The listing builds one solid part. Answer for the finished solid, in the listing's coordinates (mm). Give positions to 0.01 mm unless a question says otherwise; leave off trailing zeros. Loops run counter-clockwise (first coordinate to the right, second up) from the corner with the lowest first, then second, coordinate; pieces in that order, holes last.
Item 1: Consider line 1 along X through (y, z) = (-1.8, 37.5); line 2 along X through (y, z) = (1.7, 82.5); line 3 along Y through (x, z) = (-0.25, 95.5). Determine where each line is inside the solid, lowest interval first.
Item 2: Section A-A, the plane z = 97.5 is taken. Give the vertices of the cut face in (x, y).
Item 3: Section B-B, the plane z = 19 is taken. Give the vertices of the cut face in (x, y).
Item 4: Section C-C, the plane x = 0 is taken. Give the number of separate pieces and of enclosed holes in the cut face, and give its area (3 significant figures).
Item 5: This flat-tipped pin is pushed along its axis until it touches: pin 1 Ø2 at (x, z) = (0.5, 53) entering from +Y. Where does it stop, or does it pass through?
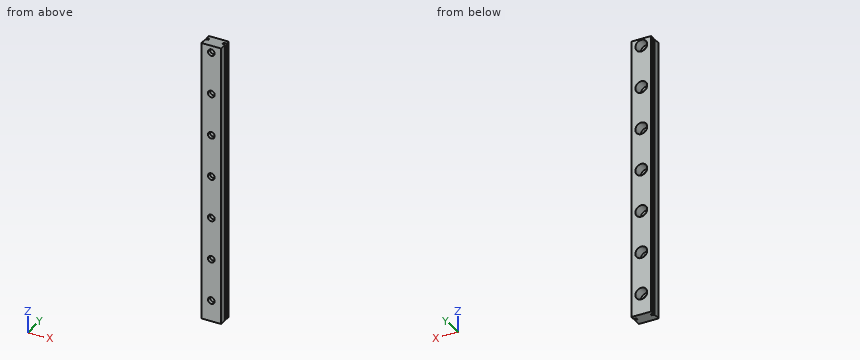
from build123d import *

# Parameters (mm, degrees)
SKETCH_1_W          = 7
SKETCH_1_H          = 4.8
EXTRUDE_1_DEPTH     = 100
SKETCH_2_R          = 1.2
CUT_EXTRUDE_1_DEPTH = 5.8
SKETCH_3_R          = 2.1
CUT_EXTRUDE_2_DEPTH = 3.5
CUT_EXTRUDE_3_DEPTH = 101


with BuildPart() as part:
    # 草图1 → 凸台-拉伸1 (new body)
    with BuildSketch(Plane.XY):
        Rectangle(SKETCH_1_W, SKETCH_1_H)
    extrude(amount=EXTRUDE_1_DEPTH)

    # 草图2 → 切除-拉伸1 (cut, through all)
    with BuildSketch(Plane(origin=(0, 2.4, 0), x_dir=(1, 0, 0), z_dir=(0, 1, 0))):
        with Locations((0, -7.5)):
            Circle(SKETCH_2_R)
        with Locations((0, -22.5)):
            Circle(SKETCH_2_R)
        with Locations((0, -37.5)):
            Circle(SKETCH_2_R)
        with Locations((0, -52.5)):
            Circle(SKETCH_2_R)
        with Locations((0, -67.5)):
            Circle(SKETCH_2_R)
        with Locations((0, -82.5)):
            Circle(SKETCH_2_R)
        with Locations((0, -97.5)):
            Circle(SKETCH_2_R)
        with Locations((0, -112.5)):
            Circle(SKETCH_2_R)
        with Locations((0, -127.5)):
            Circle(SKETCH_2_R)
        with Locations((0, -142.5)):
            Circle(SKETCH_2_R)
        with Locations((0, -157.5)):
            Circle(SKETCH_2_R)
        with Locations((0, -172.5)):
            Circle(SKETCH_2_R)
        with Locations((0, -187.5)):
            Circle(SKETCH_2_R)
        with Locations((0, -202.5)):
            Circle(SKETCH_2_R)
        with Locations((0, -217.5)):
            Circle(SKETCH_2_R)
        with Locations((0, -232.5)):
            Circle(SKETCH_2_R)
        with Locations((0, -247.5)):
            Circle(SKETCH_2_R)
        with Locations((0, -262.5)):
            Circle(SKETCH_2_R)
        with Locations((0, -277.5)):
            Circle(SKETCH_2_R)
        with Locations((0, -292.5)):
            Circle(SKETCH_2_R)
    extrude(amount=-CUT_EXTRUDE_1_DEPTH, mode=Mode.SUBTRACT)

    # 草图3 → 切除-拉伸2 (cut)
    with BuildSketch(Plane(origin=(0, 2.4, 0), x_dir=(1, 0, 0), z_dir=(0, 1, 0))):
        with Locations((0, -7.5)):
            Circle(SKETCH_3_R)
        with Locations((0, -22.5)):
            Circle(SKETCH_3_R)
        with Locations((0, -37.5)):
            Circle(SKETCH_3_R)
        with Locations((0, -52.5)):
            Circle(SKETCH_3_R)
        with Locations((0, -67.5)):
            Circle(SKETCH_3_R)
        with Locations((0, -82.5)):
            Circle(SKETCH_3_R)
        with Locations((0, -97.5)):
            Circle(SKETCH_3_R)
        with Locations((0, -112.5)):
            Circle(SKETCH_3_R)
        with Locations((0, -127.5)):
            Circle(SKETCH_3_R)
        with Locations((0, -142.5)):
            Circle(SKETCH_3_R)
        with Locations((0, -157.5)):
            Circle(SKETCH_3_R)
        with Locations((0, -172.5)):
            Circle(SKETCH_3_R)
        with Locations((0, -187.5)):
            Circle(SKETCH_3_R)
        with Locations((0, -202.5)):
            Circle(SKETCH_3_R)
        with Locations((0, -217.5)):
            Circle(SKETCH_3_R)
        with Locations((0, -232.5)):
            Circle(SKETCH_3_R)
        with Locations((0, -247.5)):
            Circle(SKETCH_3_R)
        with Locations((0, -262.5)):
            Circle(SKETCH_3_R)
        with Locations((0, -277.5)):
            Circle(SKETCH_3_R)
        with Locations((0, -292.5)):
            Circle(SKETCH_3_R)
    extrude(amount=-CUT_EXTRUDE_2_DEPTH, mode=Mode.SUBTRACT)

    # 草图4 → 切除-拉伸3 (cut, through all)
    with BuildSketch(Plane(origin=(0, 0, 0), x_dir=(-1, 0, 0), z_dir=(0, 0, -1))):
        Polygon((3.5, 1.1), (2.5, 0.9), (2.5, 0.3), (3.5, 0.1), align=None)
        Polygon((-3.5, 1.1), (-2.5, 0.9), (-2.5, 0.3), (-3.5, 0.1), align=None)
    extrude(amount=-CUT_EXTRUDE_3_DEPTH, mode=Mode.SUBTRACT)


solid = part.part
Worked answers:
1. line 1: x = -3.5 to -1.2, 1.2 to 3.5
1. line 2: x = -3.5 to -2.1, 2.1 to 3.5
1. line 3: y = -2.4 to -1.1
2. outline: (-3.5, -2.4) - (-1.2, -2.4) - (-1.2, -1.1) - (-2.1, -1.1) - (-2.1, 2.4) - (-3.5, 2.4) - (-3.5, 1.1) - (-2.5, 0.9) - (-2.5, 0.3) - (-3.5, 0.1) - close; (1.2, -2.4) - (3.5, -2.4) - (3.5, 0.1) - (2.5, 0.3) - (2.5, 0.9) - (3.5, 1.1) - (3.5, 2.4) - (2.1, 2.4) - (2.1, -1.1) - (1.2, -1.1) - close
3. outline: (-3.5, -2.4) - (3.5, -2.4) - (3.5, 0.1) - (2.5, 0.3) - (2.5, 0.9) - (3.5, 1.1) - (3.5, 2.4) - (-3.5, 2.4) - (-3.5, 1.1) - (-2.5, 0.9) - (-2.5, 0.3) - (-3.5, 0.1) - close
4. separate pieces: 8
4. enclosed holes: 0
4. area: 355 mm2
5. pin 1: stops at y = -1.1
